```python
from build123d import *

# Parameters (mm, degrees)
EXTRUDE_1_DEPTH     = 3
EXTRUDE_START       = -3
EXTRUDE_2_DEPTH     = 3
EXTRUDE_3_DEPTH     = 3
SKETCH_4_R          = 2.187098749
CUT_EXTRUDE_1_DEPTH = 10
SKETCH_5_R          = 1.75
CUT_EXTRUDE_2_DEPTH = 10


with BuildPart() as part:
    # 草图1 → 凸台-拉伸1 (new body)
    with BuildSketch(Plane.XY):
        with BuildLine():
            Line((-34.464101615, 23.287401575), (34.464101615, 23.287401575))
            ThreePointArc((34.464101615, 23.287401575), (34.981739705, 23.219253227), (35.464101615, 23.019452382))
            Line((35.464101615, 23.019452382), (54.167481352, 12.221051057))
            ThreePointArc((54.167481352, 12.221051057), (54.899532159, 11.489000249), (55.167481352, 10.489000249))
            Line((55.167481352, 10.489000249), (55.167481352, -10.489000249))
            ThreePointArc((55.167481352, -10.489000249), (54.899532159, -11.489000249), (54.167481352, -12.221051057))
            Line((54.167481352, -12.221051057), (35.464101615, -23.019452382))
            ThreePointArc((35.464101615, -23.019452382), (34.981739705, -23.219253227), (34.464101615, -23.287401575))
            Line((34.464101615, -23.287401575), (-34.464101615, -23.287401575))
            ThreePointArc((-34.464101615, -23.287401575), (-34.981739705, -23.219253227), (-35.464101615, -23.019452382))
            Line((-35.464101615, -23.019452382), (-54.167481352, -12.221051057))
            ThreePointArc((-54.167481352, -12.221051057), (-54.899532159, -11.489000249), (-55.167481352, -10.489000249))
            Line((-55.167481352, -10.489000249), (-55.167481352, 10.489000249))
            ThreePointArc((-55.167481352, 10.489000249), (-54.899532159, 11.489000249), (-54.167481352, 12.221051057))
            Line((-54.167481352, 12.221051057), (-35.464101615, 23.019452382))
            ThreePointArc((-35.464101615, 23.019452382), (-34.981739705, 23.219253227), (-34.464101615, 23.287401575))
        make_face()
    extrude(amount=EXTRUDE_1_DEPTH)

    # 草图2 → 凸台-拉伸2 (add)
    with BuildSketch(Plane.XY.offset(3).offset(EXTRUDE_START)):
        with BuildLine():
            Line((-55.167481352, 15.551379934), (-55.167481352, 10.489000249))
            Line((-55.167481352, 10.489000249), (-55.167481352, -10.489000249))
            ThreePointArc((-55.167481352, -10.489000249), (-54.899532159, -11.489000249), (-54.167481352, -12.221051057))
            Line((-54.167481352, -12.221051057), (-35.464101615, -23.019452382))
            ThreePointArc((-35.464101615, -23.019452382), (-34.981739705, -23.219253227), (-34.464101615, -23.287401575))
            Line((-34.464101615, -23.287401575), (34.464101615, -23.287401575))
            ThreePointArc((34.464101615, -23.287401575), (34.981739705, -23.219253227), (35.464101615, -23.019452382))
            Line((35.464101615, -23.019452382), (54.167481352, -12.221051057))
            ThreePointArc((54.167481352, -12.221051057), (54.899532159, -11.489000249), (55.167481352, -10.489000249))
            Line((55.167481352, -10.489000249), (55.167481352, 10.489000249))
            Line((55.167481352, 10.489000249), (55.167481352, 15.551379934))
            Line((55.167481352, 15.551379934), (55.167481352, 36.529380432))
            ThreePointArc((55.167481352, 36.529380432), (54.899532159, 37.529380432), (54.167481352, 38.26143124))
            Line((54.167481352, 38.26143124), (35.464101615, 49.059832565))
            ThreePointArc((35.464101615, 49.059832565), (34.981739705, 49.25963341), (34.464101615, 49.327781758))
            Line((34.464101615, 49.327781758), (-34.464101615, 49.327781758))
            ThreePointArc((-34.464101615, 49.327781758), (-34.981739705, 49.25963341), (-35.464101615, 49.059832565))
            Line((-35.464101615, 49.059832565), (-54.167481352, 38.26143124))
            ThreePointArc((-54.167481352, 38.26143124), (-54.899532159, 37.529380432), (-55.167481352, 36.529380432))
            Line((-55.167481352, 36.529380432), (-55.167481352, 15.551379934))
        make_face()
    extrude(amount=EXTRUDE_2_DEPTH)

    # 草图3 → 凸台-拉伸3 (add)
    with BuildSketch(Plane.XY.offset(3)):
        with BuildLine():
            Line((55.167481352, 33.186292179), (-55.167481352, 33.186292179))
            Line((-55.167481352, 33.186292179), (-55.167481352, 47.90257896))
            ThreePointArc((-55.167481352, 47.90257896), (-54.899532159, 48.90257896), (-54.167481352, 49.634629768))
            Line((-54.167481352, 49.634629768), (-35.464101615, 60.433031094))
            ThreePointArc((-35.464101615, 60.433031094), (-34.981739705, 60.632831939), (-34.464101615, 60.700980286))
            Line((-34.464101615, 60.700980286), (34.464101615, 60.700980286))
            ThreePointArc((34.464101615, 60.700980286), (34.981739705, 60.632831939), (35.464101615, 60.433031094))
            Line((35.464101615, 60.433031094), (54.167481352, 49.634629768))
            ThreePointArc((54.167481352, 49.634629768), (54.899532159, 48.90257896), (55.167481352, 47.90257896))
            Line((55.167481352, 47.90257896), (55.167481352, 33.186292179))
        make_face()
    extrude(amount=-EXTRUDE_3_DEPTH)

    # 草图4 → 切除-拉伸1 (cut)
    with BuildSketch(Plane.XY.offset(3)):
        with Locations((-20.424577197, 55.161880556)):
            Circle(SKETCH_4_R)
        with Locations((19.655486733, 55.22184421)):
            Circle(SKETCH_4_R)
        with Locations((27.658697285, -14.95988945)):
            Circle(SKETCH_4_R)
        with Locations((-28.447724115, -14.95988945)):
            Circle(SKETCH_4_R)
    extrude(amount=-CUT_EXTRUDE_1_DEPTH, mode=Mode.SUBTRACT)

    # 草图5 → 切除-拉伸2 (cut)
    with BuildSketch(Plane.XY.offset(3)):
        with Locations((46.798601885, 47.255616016)):
            Circle(SKETCH_5_R)
        with Locations((-46.798601885, 47.255616016)):
            Circle(SKETCH_5_R)
        with Locations((46.798601885, -9.842037304)):
            Circle(SKETCH_5_R)
        with Locations((-46.798601885, -9.842037304)):
            Circle(SKETCH_5_R)
    extrude(amount=-CUT_EXTRUDE_2_DEPTH, mode=Mode.SUBTRACT)


solid = part.part
```
Check sheet for the modelled part. Datum: model origin and axes. Units: mm. Give positions to 0.01 mm unless a question says otherwise; leave off trailing zeros. Write each loop counter-clockwise with the first axis right and the second up, starting at its lowest first coordinate (ties: lowest second). Pieces come first, ordered by that corner, then holes.
Item 1: Cross-section at B-B (z = 2.45). Count the separate pieces of the cut face and the enclosed holes in it, and give its area (3 significant figures).
Item 2: Draft check along Y on faces 1 (the face through (0, -23.287, 1)), 2 (the face through (45.51, 48.44, 1.52)), 3 (the face through (-19.42, 53.22, 1.52)), 4 (the face through (55.167, 19, 1)). Enter one of: released by +Y, released by -Y, zero draft, split by the parting line, or undercut.
Item 3: Scan lines: L1, parallel to X at y = 47, z = 1.6; L2, parallel to X at y = 46, z = 2; L3, parallel to Y at x = 27, z = 2.85. Record each from-to range of solid material in increasing order.
Item 4: Cross-section at A-A (x = -20). Enter the section's corners in (y, z), and give its area (3 significant figures).
Report:
1. separate pieces: 1
1. enclosed holes: 8
1. area: 8,700 mm2
2. face 1: released by -Y
2. face 2: undercut
2. face 3: undercut
2. face 4: zero draft
3. L1: x = -55.17 to -48.53, -45.07 to 45.07, 48.53 to 55.17
3. L2: x = -55.17 to -48.02, -45.58 to 45.58, 48.02 to 55.17
3. L3: y = -23.29 to -17.05, -12.87 to 60.7
4. outline: (-23.29, 0) - (53.02, 0) - (53.02, 3) - (-23.29, 3) - close; (57.31, 0) - (60.7, 0) - (60.7, 3) - (57.31, 3) - close
4. area: 239 mm2
